Input: dimensioned drawing with shaded views. Units: mm. Origin: part minimum x, y, z. A direction names the side the tool comes from. Give positions to 0.01 mm unless a question says otherwise; leave off trailing zeros. Write each loop counter-clockwise with the first axis right and the second up, starting at its lowest first coordinate (ties: lowest second). Pieces come first, ordered by that corner, then holes. Notation, with made-up numbers: (83, 66.25) -> (122, 66.25) arc R29 cw to (122, 99.25) -> close; hole circle Ø11 at (-27, -23). An arc over 180 degrees is marked (long way). Answer as a JSON object with one key per item and string values. Group by question number.
(1) Section query A-A on y = 4.5. Output: boundary loops of the cut face in (x, z).
(2) Set-up query: the marked faces 4, 5 and 6. Return all of +Z, -Z, +X, -X, +Y, -Y with unobstructed straight access to the full face (end or side cutting, diameter ignored); none if empty.
(3) Draft query along Y for the marked faces 1, 2 and 3. Return one class per face: +Y half, -Y half, draft (parallel to the pull), parting line (faces both ways), or undercut.
(4) Section query D-D on y = 17. Output: boundary loops of the cut face in (x, z).
(5) Section query C-C on x = 11.5. Output: boundary loops of the cut face in (y, z).
(6) Section query B-B on z = 17. Output: boundary loops of the cut face in (x, y) (3 decimals).
(7) Material intervals for probe 1 along Y at (x, z) = (49.5, 25) (3 decimals); probe 2 along Z at (x, y) = (46, 10); probe 3 along X at (y, z) = (46, 23.5), sorted ascending.
(8) Contact query for flat-ended pins moving along their axis: pin 1 Ø1 at (x, y) = (41, 27) entering from +Z; pin 2 Ø8 at (y, z) = (16, 31) entering from -X; pin 3 Ø14 at (y, z) = (41.5, 20) entering from -X; pin 4 Ø6.5 at (x, z) = (40, 17.5) entering from -Y. Output: stop coordinate, or through.
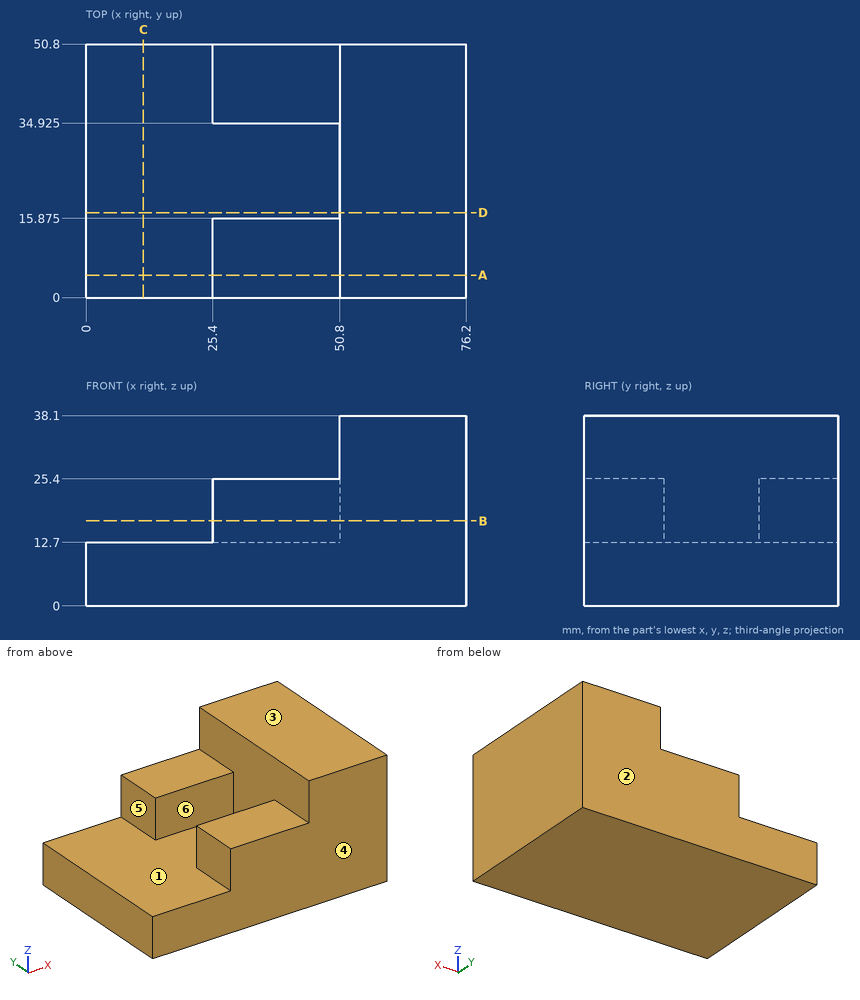
Answer list:
{
 "1": {"outline": "(0, 0) -> (76.2, 0) -> (76.2, 38.1) -> (50.8, 38.1) -> (50.8, 25.4) -> (25.4, 25.4) -> (25.4, 12.7) -> (0, 12.7) -> close"},
 "2": {"face 4": "+Z, -Z, +X, -X, -Y", "face 5": "+Z, -X, +Y, -Y", "face 6": "+Z, -X"},
 "3": {"face 1": "undercut", "face 2": "+Y half", "face 3": "draft"},
 "4": {"outline": "(0, 0) -> (76.2, 0) -> (76.2, 38.1) -> (50.8, 38.1) -> (50.8, 12.7) -> (0, 12.7) -> close"},
 "5": {"outline": "(0, 0) -> (50.8, 0) -> (50.8, 12.7) -> (0, 12.7) -> close"},
 "6": {"outline": "(25.4, 0) -> (76.2, 0) -> (76.2, 50.8) -> (25.4, 50.8) -> (25.4, 34.925) -> (50.8, 34.925) -> (50.8, 15.875) -> (25.4, 15.875) -> close"},
 "7": {"probe 1": "0 to 15.875, 34.925 to 50.8", "probe 2": "0 to 25.4", "probe 3": "25.4 to 76.2"},
 "8": {"pin 1": "z = 12.7", "pin 2": "x = 50.8", "pin 3": "x = 25.4", "pin 4": "y = 0"}
}
